Can you work these out from the model? Positions are in its coordinate system, mm. A direction names the side the tool comes from. Round coordinates to 2 decimals unless told otherwise and drop trailing zeros. Order: outer loops, then holes, each group sorted by start corner. A loop starts at its lowest first (then second) coordinate and runs counter-clockwise, first axis right, second up. Notation, with made-up numbers: M 44,13 L 94,13 A25 ccw 94,35 Z; hole C -16.5,-27 d2. An arc over 180 degrees is marked long. One line per question, with ' | ' between items.
```python
from build123d import *

# Parameters (mm, degrees)
BOSS_EXTRUDE1_DEPTH = 1.3
SKETCH2_R           = 2.35
CUT_EXTRUDE1_DEPTH  = 1.3
SKETCH3_R           = 3.4
SKETCH3_R_2         = 2.35
BOSS_EXTRUDE2_DEPTH = 2.5
BOSS_EXTRUDE3_START = -1.1
SKETCH4_R           = 2.35
SKETCH4_R_2         = 2.1
BOSS_EXTRUDE3_DEPTH = 0.6
CUT_EXTRUDE3_REACH  = 5.8
SKETCH5_R           = 0.5


with BuildPart() as part:
    # Sketch1 → Boss-Extrude1 (new body)
    with BuildSketch(Plane.XY):
        with BuildLine():
            Line((13, 1.8), (2.304343724, 2.5))
            ThreePointArc((2.304343724, 2.5), (-3.4, 0), (2.304343724, -2.5))
            Line((2.304343724, -2.5), (13, -1.8))
            ThreePointArc((13, -1.8), (14.8, 0), (13, 1.8))
        make_face()
    extrude(amount=BOSS_EXTRUDE1_DEPTH)

    # Sketch2 → Cut-Extrude1 (cut)
    with BuildSketch(Plane.XY.offset(1.3)):
        Circle(SKETCH2_R)
    extrude(amount=-CUT_EXTRUDE1_DEPTH, mode=Mode.SUBTRACT)

    # Sketch3 → Boss-Extrude2 (add)
    with BuildSketch(Plane.XY.offset(1.3)):
        Circle(SKETCH3_R)
        Circle(SKETCH3_R_2, mode=Mode.SUBTRACT)
    extrude(amount=BOSS_EXTRUDE2_DEPTH)

    # Sketch4 → Boss-Extrude3 (add)
    with BuildSketch(Plane(origin=(0, 0, 0), x_dir=(-1, 0, 0), z_dir=(0, 0, -1)).offset(BOSS_EXTRUDE3_START)):
        Circle(SKETCH4_R)
        Circle(SKETCH4_R_2, mode=Mode.SUBTRACT)
    extrude(amount=-BOSS_EXTRUDE3_DEPTH)

    # Sketch5 → Cut-Extrude3 (cut, up to next)
    with BuildSketch(Plane(origin=(0, 0, 0), x_dir=(-1, 0, 0), z_dir=(0, 0, -1)), mode=Mode.PRIVATE) as cut_extrude3_sk1:
        with Locations((-13, 0)):
            Circle(SKETCH5_R)
    cut_extrude3_tool1 = extrude(cut_extrude3_sk1.sketch, amount=-CUT_EXTRUDE3_REACH, mode=Mode.PRIVATE) & part.part
    add(cut_extrude3_tool1.solids().sort_by_distance((13, 0, 0))[0], mode=Mode.SUBTRACT)
    # Sketch5 → Cut-Extrude3 (cut, up to next)
    with BuildSketch(Plane(origin=(0, 0, 0), x_dir=(-1, 0, 0), z_dir=(0, 0, -1)), mode=Mode.PRIVATE) as cut_extrude3_sk2:
        with Locations((-11.25, 0)):
            Circle(SKETCH5_R)
    cut_extrude3_tool2 = extrude(cut_extrude3_sk2.sketch, amount=-CUT_EXTRUDE3_REACH, mode=Mode.PRIVATE) & part.part
    add(cut_extrude3_tool2.solids().sort_by_distance((11.25, 0, 0))[0], mode=Mode.SUBTRACT)
    # Sketch5 → Cut-Extrude3 (cut, up to next)
    with BuildSketch(Plane(origin=(0, 0, 0), x_dir=(-1, 0, 0), z_dir=(0, 0, -1)), mode=Mode.PRIVATE) as cut_extrude3_sk3:
        with Locations((-9.5, 0)):
            Circle(SKETCH5_R)
    cut_extrude3_tool3 = extrude(cut_extrude3_sk3.sketch, amount=-CUT_EXTRUDE3_REACH, mode=Mode.PRIVATE) & part.part
    add(cut_extrude3_tool3.solids().sort_by_distance((9.5, 0, 0))[0], mode=Mode.SUBTRACT)
    # Sketch5 → Cut-Extrude3 (cut, up to next)
    with BuildSketch(Plane(origin=(0, 0, 0), x_dir=(-1, 0, 0), z_dir=(0, 0, -1)), mode=Mode.PRIVATE) as cut_extrude3_sk4:
        with Locations((-7.75, 0)):
            Circle(SKETCH5_R)
    cut_extrude3_tool4 = extrude(cut_extrude3_sk4.sketch, amount=-CUT_EXTRUDE3_REACH, mode=Mode.PRIVATE) & part.part
    add(cut_extrude3_tool4.solids().sort_by_distance((7.75, 0, 0))[0], mode=Mode.SUBTRACT)
    # Sketch5 → Cut-Extrude3 (cut, up to next)
    with BuildSketch(Plane(origin=(0, 0, 0), x_dir=(-1, 0, 0), z_dir=(0, 0, -1)), mode=Mode.PRIVATE) as cut_extrude3_sk5:
        with Locations((-6, 0)):
            Circle(SKETCH5_R)
    cut_extrude3_tool5 = extrude(cut_extrude3_sk5.sketch, amount=-CUT_EXTRUDE3_REACH, mode=Mode.PRIVATE) & part.part
    add(cut_extrude3_tool5.solids().sort_by_distance((6, 0, 0))[0], mode=Mode.SUBTRACT)
    # Sketch5 → Cut-Extrude3 (cut, up to next)
    with BuildSketch(Plane(origin=(0, 0, 0), x_dir=(-1, 0, 0), z_dir=(0, 0, -1)), mode=Mode.PRIVATE) as cut_extrude3_sk6:
        with Locations((-4.25, 0)):
            Circle(SKETCH5_R)
    cut_extrude3_tool6 = extrude(cut_extrude3_sk6.sketch, amount=-CUT_EXTRUDE3_REACH, mode=Mode.PRIVATE) & part.part
    add(cut_extrude3_tool6.solids().sort_by_distance((4.25, 0, 0))[0], mode=Mode.SUBTRACT)


solid = part.part
```
(1) Will these pins go through, and if not, where does the flat tip stop? pin 1 Ø1.4 at (x, y) = (0, -0.5) entering from -Z; pin 2 Ø4 at (x, y) = (8, 0.5) entering from +Z; pin 3 Ø1 at (y, z) = (-1.5, 1) entering from +X; pin 4 Ø4 at (x, y) = (8.5, 0) entering from -Z.
Final values:
pin 1: through | pin 2: z = 1.3 | pin 3: x = 14.5 | pin 4: z = 0
(2) If we section it at D-D on x = 4: Please give me the cut outline in (y, z), plus the area to 3 significant figures.
Final values:
outline: M -2.39,0 L -0.43,0 L -0.43,1.3 L -2.39,1.3 Z; M 0.43,0 L 2.39,0 L 2.39,1.3 L 0.43,1.3 Z | area: 5.09 mm^2
(3) Thinking about a two-plate mould opening in X: for faces 3 (the cylindrical face through (-0.509, -2.294, 2.735)), 4 (the flat face through (6, -1, 0)), 5 (the flat face through (7.577, -2.155, 0.641)), which applies, released by +X, released by -X, zero draft, split by the parting line, or undercut?
Final values:
face 3: undercut | face 4: zero draft | face 5: released by +X
(4) If we section it at A-A on x = 9.25: Please give me the cut outline in (y, z).
Final values:
outline: M -2.05,0 L -0.43,0 L -0.43,1.3 L -2.05,1.3 Z; M 0.43,0 L 2.05,0 L 2.05,1.3 L 0.43,1.3 Z
(5) If we section it at C-C on z = 2.85: Please give me the cut outline in (x, y).
Final values:
outline: C 0,0 d6.8; hole C 0,0 d4.7
(6) On a 3-axis mill with a long thin cutter (end or side, diameter ignored), from which of +Z, -Z, +X, -X, +Y, -Y can I reach the whole of each face in a straight line? I mean faces 1 (the cylindrical face through (-0.509, -2.294, 0.542)), 2 (the cylindrical face through (14.8, 0, 0.6)). Say none if no direction works.
Final values:
face 1: -Z | face 2: +Z, -Z, +X
(7) Please list where these lines run through material, in increasing order: probe 1 along Y at (x, z) = (0, 1.5); probe 2 along Y at (x, z) = (6, 0.35); probe 3 along X at (y, z) = (0.25, 2.7). Write a range as [from, to].
Final values:
probe 1: [-3.4, -2.1], [2.1, 3.4] | probe 2: [-2.26, -0.5], [0.5, 2.26] | probe 3: [-3.39, -2.34], [2.34, 3.39]
(8) If we section it at B-B on y = 0: State how many separate pieces and enclosed holes the cut face has, plus the area to 3 significant figures.
Final values:
separate pieces: 8 | enclosed holes: 0 | area: 15.3 mm^2
